Design review of the part built by this model. Coordinates are the model's own, in mm. Face numbers are marked on the shaded views. A direction names the side the tool comes from. Coordinates: 2 decimals unless noted, no trailing zeros. Write each loop counter-clockwise with the first axis right and the second up, starting at its lowest first coordinate (ties: lowest second). Pieces come first, ordered by that corner, then holes. Notation, with made-up numbers: (-3.75, -38) - (2.25, -38) arc R32 cw to (2.25, -6) - close; hole circle Ø10 at (79.25, 35). An arc over 180 degrees is marked (long way). Answer as a JSON object with one key per item and string values.
```python
from build123d import *

# Parameters (mm, degrees)
F2_R          = 3.175
F2_R_2        = 2.75
F3_DEPTH      = 6
F3_DEPTH_BACK = 5
F4_R          = 0.3
F5_R          = 2.75
F6_DEPTH      = 6.966563666
F8_D          = 2


with BuildPart() as f1:
    # F0 (on Front) → F1 (revolve)
    with BuildSketch(Plane.XZ):
        Polygon((0, 2), (0, 0), (30, 0), (30, 2), (17.0486500744, 2), align=None)
        with BuildLine():
            ThreePointArc((17.0486500744, 6.965563649), (8.8785315808, 3.2666573852), (1.21e-08, 2))
            Line((1.21e-08, 2), (17.0486500744, 2))
            Line((17.0486500744, 2), (17.0486500744, 6.965563649))
        make_face()
    revolve(axis=Axis((0, 0, 32.75), (0, 0, -1)))

    # F2 (on Top) → F3 (join, two sides)
    with BuildSketch(Plane.XY) as f3_sk:
        Circle(F2_R)
        Circle(F2_R_2, mode=Mode.SUBTRACT)
    extrude(amount=F3_DEPTH)
    extrude(f3_sk.sketch, amount=-F3_DEPTH_BACK)

    # F4
    f4_edges = [f1.edges().sort_by_distance(p)[0] for p in [
        (-3.175, 0, 6),
    ]]
    fillet(f4_edges, radius=F4_R)

    # F5 (on face) → F6 (cut, through all)
    with BuildSketch(Plane(origin=(0, 0, 0), x_dir=(1, 0, 0), z_dir=(0, 0, -1))):
        Circle(F5_R)
    extrude(amount=-F6_DEPTH, mode=Mode.SUBTRACT)

    # F8 (through all)
    with Locations(Plane(origin=(0, 0, 0), x_dir=(1, 0, 0), z_dir=(0, 0, -1))):
        with Locations((-6.175, 0), (6.175, 0)):
            Hole(F8_D / 2)


solid = f1.part
```
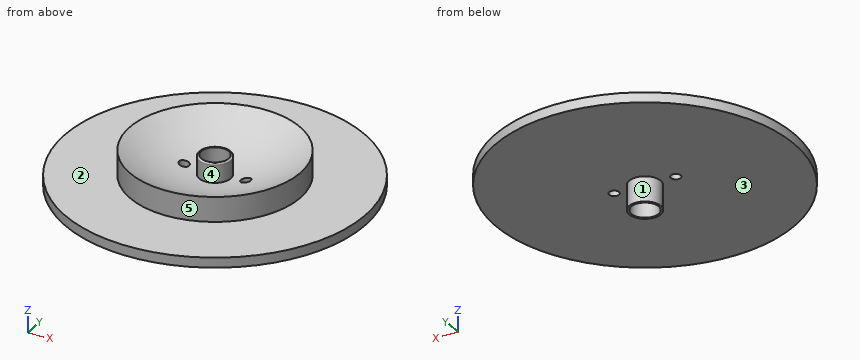
(1) Tool access review of the marked faces 1 and 2: name each direction out of +Z, -Z, +X, -X, +Y, -Y from which nothing blocks a thin tool from reaching the whole face with its end or side.
Solved:
{"face 1": "-Z", "face 2": "+Z"}
(2) Take a section at C-C, the plane y = -6. Write out the cut boundary in (x, z).
Solved:
{"outline": "(-29.39, 0) - (29.39, 0) - (29.39, 2) - (15.96, 2) - (15.96, 6.97) arc R31.18 cw to (-15.96, 6.97) - (-15.96, 2) - (-29.39, 2) - close"}
(3) For pin 1 (3.5 mm diameter, centred on x = 0, y = 0, fed in from -Z); pin 2 (1 mm diameter, centred on x = 19.5, y = -12, fed in from -Z); pin 3 (18 mm diameter, centred on x = 1.5, y = -3, fed in from +Z); pin 4 (2.5 mm diameter, centred on x = -6.175, y = 0, fed in from +Z), all flat-tipped, find the tip position at first contact; note any pin that passes through.
Solved:
{"pin 1": "passes through", "pin 2": "stops at z = 0", "pin 3": "stops at z = 6", "pin 4": "stops at z = 2.88"}
(4) Take a section at D-D, the plane y = 0. Give the number of separate pieces and of enclosed holes in the cut face, and give its area (3 significant figures).
Solved:
{"separate pieces": "4", "enclosed holes": "0", "area": "160 mm^2"}
(5) To check wall thickness, follow line 1 (X direction, y = 0, z = 4.8) (3 decimals); line 2 (Y direction, x = 0, z = 4.65) (3 decimals); line 3 (X direction, y = 2.5, z = 5). State the ranges of each line that lie inside material, in increasing order. Write a range as from..to.
Solved:
{"line 1": "x = -17.049..-13.037, -3.175..-2.75, 2.75..3.175, 13.037..17.049", "line 2": "y = -17.049..-12.699, -3.175..-2.75, 2.75..3.175, 12.699..17.049", "line 3": "x = -16.86..-13.24, -1.96..-1.15, 1.15..1.96, 13.24..16.86"}
(6) The part is to be moulded in two halves that separate along Y. For the marked faces 3, 4 and 5, say which applies: pulls with the +Y half, pulls with the -Y half, needs draft (parallel to the pull), parting line crosses it, or undercut.
Solved:
{"face 3": "needs draft", "face 4": "undercut", "face 5": "parting line crosses it"}
(7) Take a section at B-B, the plane z = -3. Write out the cut boundary in (x, y) (3 decimals).
Solved:
{"outline": "circle Ø6.35 at (0, 0); hole circle Ø5.5 at (0, 0)"}
(8) Take a section at A-A, the plane x = 0. Write out the cut boundary in (y, z) (3 decimals).
Solved:
{"outline": "(-30, 0) - (-3.175, 0) - (-3.175, -5) - (-2.75, -5) - (-2.75, 6) - (-2.875, 6) arc R0.3 ccw to (-3.175, 5.7) - (-3.175, 2.159) arc R31.75 cw to (-17.049, 6.966) - (-17.049, 2) - (-30, 2) - close; (2.75, -5) - (3.175, -5) - (3.175, 0) - (30, 0) - (30, 2) - (17.049, 2) - (17.049, 6.966) arc R31.75 cw to (3.175, 2.159) - (3.175, 5.7) arc R0.3 ccw to (2.875, 6) - (2.75, 6) - close"}
